```python
from build123d import *

# Parameters (mm, degrees)
F1_DEPTH = 1.5
F2_R     = 3
F3_R     = 2.4
F4_R     = 0.99999
F5_R     = 8


# Not quite as in the source:
# - a fillet or chamfer is up to 0.001 mm smaller than in the source, because OpenCascade refuses the exact size


with BuildPart() as f1:
    # F0 (on Top) → F1 (new body)
    with BuildSketch(Plane.XY):
        with BuildLine():
            ThreePointArc((-7.2162480919, 3.2149282225), (1.6434171829, 7.7271715371), (7.9, 0))
            Line((7.9, 0), (7.9, 29.9))
            Line((7.9, 29.9), (2.9, 29.9))
            Line((2.9, 29.9), (-7.2162480919, 3.2149282225))
        make_face()
        with BuildLine():
            Line((2.9, 29.9), (7.9, 29.9))
            Line((7.9, 29.9), (12.9, 29.9))
            ThreePointArc((12.9, 29.9), (28.5747012766, 11.2865794971), (31.9942384958, -12.8062088042))
            Line((31.9942384958, -12.8062088042), (36.9942384958, -12.8062088042))
            ThreePointArc((36.9942384958, -12.8062088042), (32.2218442931, 14.721028685), (12.9, 34.9))
            ThreePointArc((12.9, 34.9), (6.9234468079, 34.3531063842), (2.9, 29.9))
        make_face()
        with BuildLine():
            ThreePointArc((5.9, 0), (5.4508892418, -2.257832251), (4.171930009, -4.171930009))
            Line((4.171930009, -4.171930009), (5.5861435714, -5.5861435714))
            ThreePointArc((5.5861435714, -5.5861435714), (7.2986483068, -3.0231991157), (7.9, 0))
            ThreePointArc((7.9, 0), (1.6434171829, 7.7271715371), (-7.2162480919, 3.2149282225))
            ThreePointArc((-7.2162480919, 3.2149282225), (-7.7678841556, -1.4387410276), (-5.5861435714, -5.5861435714))
            Line((-5.5861435714, -5.5861435714), (-4.171930009, -4.171930009))
            ThreePointArc((-4.171930009, -4.171930009), (-2.257832251, 5.4508892418), (5.9, 0))
        make_face()
    extrude(amount=F1_DEPTH)

    # F2
    f2_edges = [f1.edges().sort_by_distance(p)[0] for p in [
        (7.9, 29.9, 0.75),
        (12.9, 29.9, 0.75),
    ]]
    fillet(f2_edges, radius=F2_R)

    # F3
    f3_edges = [f1.edges().sort_by_distance(p)[0] for p in [
        (31.994238, -12.806209, 0.75),
        (36.994238, -12.806209, 0.75),
    ]]
    fillet(f3_edges, radius=F3_R)

    # F4 (radius 1 in the source; OpenCascade refuses exactly that, so slightly less here)
    f4_edges = [f1.edges().sort_by_distance(p)[0] for p in [
        (4.17193, -4.17193, 0.75),
        (-4.17193, -4.17193, 0.75),
        (5.586144, -5.586144, 0.75),
        (-5.586144, -5.586144, 0.75),
    ]]
    fillet(f4_edges, radius=F4_R)

    # F5
    f5_edges = [f1.edges().sort_by_distance(p)[0] for p in [
        (12.9, 34.9, 0.75),
    ]]
    fillet(f5_edges, radius=F5_R)


solid = f1.part
```
Source: CAD feature listing. Evaluate the final solid. Frame: model axes, mm. A direction names the side the tool comes from. Coordinates: 2 decimals unless noted, no trailing zeros. Write each loop counter-clockwise with the first axis right and the second up, starting at its lowest first coordinate (ties: lowest second). Pieces come first, ordered by that corner, then holes. Notation, with made-up numbers: M 55,55 L 94,55 A12 ccw 94,64 Z; hole C -33,49.25 d11. An arc over 180 degrees is marked long. Answer as a JSON object with one key per item and string values.
1. Cut plane B-B on y = 5. Output: boundary loops of the cut face in (x, z).
Evaluation:
{"outline": "M -6.54,0 L -3.13,0 L -3.13,1.5 L -6.54,1.5 Z; M 3.13,0 L 7.9,0 L 7.9,1.5 L 3.13,1.5 Z; M 30.83,0 L 35.87,0 L 35.87,1.5 L 30.83,1.5 Z"}
2. Cut plane C-C on y = 13.5. Output: boundary loops of the cut face in (x, z).
Evaluation:
{"outline": "M -3.32,0 L 7.9,0 L 7.9,1.5 L -3.32,1.5 Z; M 27.51,0 L 32.82,0 L 32.82,1.5 L 27.51,1.5 Z"}
3. Ray query, L1, parallel to X at y = -4.5, z = 0.45; L2, parallel to X at y = 3.5, z = 0.9; L3, parallel to X at y = 15.5, z = 0.45. Return the intervals inside material, ascending.
Evaluation:
{"L1": "-6.49 to -4.61, 4.61 to 6.49, 32.36 to 37.31", "L2": "-7.11 to -4.75, 4.75 to 7.9, 31.22 to 36.23", "L3": "-2.56 to 7.9, 26.41 to 31.82"}
4. Contact query for flat-ended pins moving along their axis: P1, Ø10, axis at x = 10, y = 16, coming from the +Z side; P2, Ø0.9, axis at x = 11, z = 0.5, coming from the -Y side. Output: stop coordinate, or through.
Evaluation:
{"P1": "z = 1.5", "P2": "y = 29.88"}
5. Access query for faces 4 (the cylindrical face through (-4.538, -4.203, 0.76)), 5 (the flat face through (-2.09, 16.74, 0.74)), 6 (the flat face through (11.4, 29.9, 0.7)). Directions: +Z, -Z, +X, -X, +Y, -Y. A direction counts if a zero-diameter tool reaches every point of the face in a straight line with its end or side. Return the directions, or none.
Evaluation:
{"face 4": "+Z, -Z", "face 5": "+Z, -Z, -X, +Y", "face 6": "+Z, -Z, -Y"}
6. Cut plane A-A on y = 23. Output: boundary loops of the cut face in (x, z).
Evaluation:
{"outline": "M 0.28,0 L 7.9,0 L 7.9,1.5 L 0.28,1.5 Z; M 20.9,0 L 26.91,0 L 26.91,1.5 L 20.9,1.5 Z"}
7. Draft query along X for faces 1 (the cylindrical face through (36.44, -12.18, 0.76)), 2 (the cylindrical face through (3.12, 30.424, 0.74)), 3 (the cylindrical face through (-5.619, -5.117, 0.76)). Return one class per face: released by +X, released by -X, zero draft, split by the parting line, or undercut.
Evaluation:
{"face 1": "released by +X", "face 2": "released by -X", "face 3": "undercut"}
8. Cut plane D-D on x = -2.5. Output: boundary loops of the cut face in (y, z).
Evaluation:
{"outline": "M 5.34,0 L 15.66,0 L 15.66,1.5 L 5.34,1.5 Z"}
